from build123d import *

# Parameters (mm, degrees)
SKETCH1_W           = 382
SKETCH1_H           = 405
BOSS_EXTRUDE1_DEPTH = 2
CUT_EXTRUDE2_DEPTH  = 296.144032635


with BuildPart() as part:
    # Sketch1 → Boss-Extrude1 (new body)
    with BuildSketch(Plane(origin=(0, 0, 0), x_dir=(-1, 0, 0), z_dir=(0, 0, -1))):
        with Locations((0, 22.5)):
            Rectangle(SKETCH1_W, SKETCH1_H)
    extrude(amount=-BOSS_EXTRUDE1_DEPTH)

    # Sketch4 → Cut-Extrude2 (cut, through all)
    with BuildSketch(Plane.XY.offset(2)):
        with BuildLine():
            Line((72.225, -35.25), (-72.225, -35.25))
            ThreePointArc((-72.225, -35.25), (-87.484996723, -51.072630075), (-71.120463898, -65.75))
            Line((-71.120463898, -65.75), (71.120463898, -65.75))
            ThreePointArc((71.120463898, -65.75), (87.484996723, -51.072630075), (72.225, -35.25))
        make_face()
    extrude(amount=-CUT_EXTRUDE2_DEPTH, mode=Mode.SUBTRACT)


solid = part.part
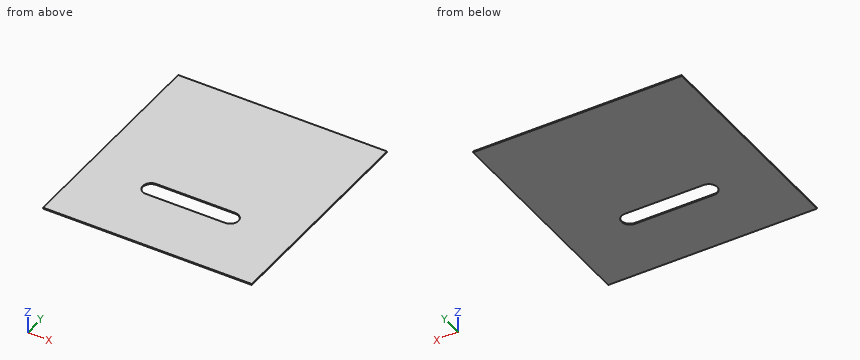
Check sheet for the modelled part. Datum: model origin and axes. Units: mm. Give positions to 0.01 mm unless a question says otherwise; leave off trailing zeros. Loops run counter-clockwise (first coordinate to the right, second up) from the corner with the lowest first, then second, coordinate; pieces in that order, holes last. Notation, with made-up numbers: M -39.75,88.5 L -17.75,88.5 A12 ccw -17.75,109.5 Z; hole C -15,62 d9. An arc over 180 degrees is marked long. Answer as a JSON object with one key per item and string values. Group by question number.
Q1. Material ranges on line 1 along Y through (x, z) = (29, 1.95); line 2 along X through (y, z) = (-60.5, 1.5); line 3 along X through (y, z) = (-58, 1.85), recorded low to high. Write a range as [from, to].
Q2. Cross-section at B-B on x = 16. Record the cut outline in (y, z).
Q3. Cross-section at A-A on y = -50.52. Record the cut outline in (x, z) (3 decimals).
Q4. Cross-section at C-C on z = 1.2. Record the cut outline in (x, y) (3 decimals).
Evaluation:
{
 "1": {"line 1": "y = [-180, -65.75], [-35.25, 225]", "line 2": "x = [-191, -83.78], [83.78, 191]", "line 3": "x = [-191, -85.54], [85.54, 191]"},
 "2": {"outline": "M -180,0 L -65.75,0 L -65.75,2 L -180,2 Z; M -35.25,0 L 225,0 L 225,2 L -35.25,2 Z"},
 "3": {"outline": "M -191,0 L -87.495,0 L -87.495,2 L -191,2 Z; M 87.495,0 L 191,0 L 191,2 L 87.495,2 Z"},
 "4": {"outline": "M -191,-180 L 191,-180 L 191,225 L -191,225 Z; hole M -72.225,-35.25 A15.27 ccw long -71.12,-65.75 L 71.12,-65.75 A15.27 ccw long 72.225,-35.25 Z"}
}
